from build123d import *

# Parameters (mm, degrees)
SKETCH1_R               = 6.5
SKETCH1_R_2             = 6
SKETCH1_R_3             = 5.3
BOSS_EXTRUDE1_DEPTH     = 2.5
CUT_EXTRUDE1_DEPTH      = 10.526279442
CIRPATTERN1_COUNT       = 24
CUT_EXTRUDE2_DEPTH      = 10.48407185
CUT_EXTRUDE2_DEPTH_BACK = 10.48407185
SKETCH4_R               = 1.05


with BuildPart() as part:
    # Sketch1 → Boss-Extrude1 (new, symmetric)
    # profile 1 of 3: a face of its own
    with BuildSketch(Plane(origin=(0, 0, 0), x_dir=(1, 0, 0), z_dir=(0, 1, 0))):
        with Locations(Location((0, 0, 0), (0, 0, 270))):
            Circle(SKETCH1_R)
        Circle(SKETCH1_R_2, mode=Mode.SUBTRACT)
    # profile 2 of 3: a face of its own
    with BuildSketch(Plane(origin=(0, 0, 0), x_dir=(1, 0, 0), z_dir=(0, 1, 0))):
        Circle(SKETCH1_R_2)
        Circle(SKETCH1_R_3, mode=Mode.SUBTRACT)
    # profile 3 of 3: a face of its own
    with BuildSketch(Plane(origin=(0, 0, 0), x_dir=(1, 0, 0), z_dir=(0, 1, 0))):
        Circle(SKETCH1_R_3)
    extrude(amount=BOSS_EXTRUDE1_DEPTH, both=True)

    # Sketch3 → Cut-Extrude1 (cut, symmetric)
    with BuildSketch(Plane(origin=(0, 0, 0), x_dir=(1, 0, 0), z_dir=(0, 1, 0))):
        with BuildLine():
            ThreePointArc((-2.097447593, 7.48155155), (-0.805034356, 6.699886195), (-0.253044756, 5.293955832))
            ThreePointArc((-0.253044756, 5.293955832), (0, 5.3), (0.253044756, 5.293955832))
            ThreePointArc((0.253044756, 5.293955832), (0.805034356, 6.699886195), (2.097447593, 7.48155155))
            ThreePointArc((2.097447593, 7.48155155), (0, 7.77), (-2.097447593, 7.48155155))
        make_face()
    cut_extrude1 = extrude(amount=CUT_EXTRUDE1_DEPTH, both=True, mode=Mode.SUBTRACT)

    # CirPattern1: Cut-Extrude1 ×24 about axis
    cirpattern1_axis = Axis((0, 0, 0), (0, 1, 0))
    for i in range(1, CIRPATTERN1_COUNT):
        add(cut_extrude1.rotate(cirpattern1_axis, i * 360 / CIRPATTERN1_COUNT), mode=Mode.SUBTRACT)

    # Sketch4 → Cut-Extrude2 (cut, two sides: drawn at the far end of the back side and taken through both)
    with BuildSketch(Plane(origin=(0, 0, 0), x_dir=(1, 0, 0), z_dir=(0, 1, 0)).offset(-CUT_EXTRUDE2_DEPTH_BACK)):
        with Locations(Location((0, 0, 0), (0, 0, 270))):
            Circle(SKETCH4_R)
    extrude(amount=CUT_EXTRUDE2_DEPTH + CUT_EXTRUDE2_DEPTH_BACK, mode=Mode.SUBTRACT)


solid = part.part
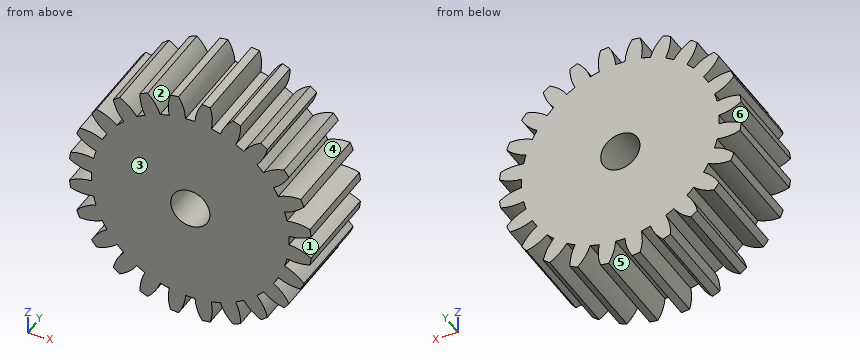
Read the model definition and answer for the solid it produces. Units are mm, in the model's axes. Face numbers are marked on the shaded views. A direction names the side the tool comes from. Round coordinates to 2 decimals unless told otherwise and drop trailing zeros. Order: outer loops, then holes, each group sorted by start corner. A loop starts at its lowest first (then second) coordinate and runs counter-clockwise, first axis right, second up.
1) The part is cut by section C-C on z = 5.5. Write down the section's boundary in (x, y), plus the area to 3 significant figures.
2) The part is cut by section A-A on z = 0. Write down the section's boundary in (x, y), plus the area to 3 significant figures.
3) The part is cut by section B-B on x = 0. Write down the section's boundary in (y, z).
4) Flat-ended cylindrical pins translate along their axes: pin 1 (1 mm diameter, centred on x = -4, y = 0.5, fed in from +Z); pin 2 (1 mm diameter, centred on y = -1, z = -1.5, fed in from +X). Find the tip coordinate at first contact, or state that the pin passes through.
5) The part is cut by section D-D on x = 5.5. Write down the section's boundary in (y, z).
6) Straight lines are drawn through the part: L1, parallel to X at y = 1.2, z = -6; L2, parallel to X at y = -1.15, z = -5; L3, parallel to Z at x = -5.5, y = 0.8. For each, find the intervals that lie inside material, in ascending order.
7) For the marked faces 4, 5 and 6, determine the directions among +Z, -Z, +X, -X, +Y, -Y from which every point of the face is accessible in a straight line to the end or side of a thin tool.
8) The mould has two halves that part along X. Classify the marked faces 1, 2 and 3: released by +X, released by -X, zero draft, split by the parting line, or undercut.
Resolved:
1. outline: (-2.67, -2.5) - (-1.81, -2.5) - (-1.81, 2.5) - (-2.67, 2.5) - close; (-1.17, -2.5) - (-0.27, -2.5) - (-0.27, 2.5) - (-1.17, 2.5) - close; (0.27, -2.5) - (1.17, -2.5) - (1.17, 2.5) - (0.27, 2.5) - close; (1.81, -2.5) - (2.67, -2.5) - (2.67, 2.5) - (1.81, 2.5) - close
1. area: 17.6 mm2
2. outline: (-5.3, -2.5) - (-1.05, -2.5) - (-1.05, 2.5) - (-5.3, 2.5) - close; (1.05, -2.5) - (5.3, -2.5) - (5.3, 2.5) - (1.05, 2.5) - close
2. area: 42.5 mm2
3. outline: (-2.5, -5.3) - (2.5, -5.3) - (2.5, -1.05) - (-2.5, -1.05) - close; (-2.5, 1.05) - (2.5, 1.05) - (2.5, 5.3) - (-2.5, 5.3) - close
4. pin 1: stops at z = 5.29
4. pin 2: stops at x = 6.42
5. outline: (-2.5, -2.67) - (2.5, -2.67) - (2.5, -1.81) - (-2.5, -1.81) - close; (-2.5, -1.17) - (2.5, -1.17) - (2.5, -0.27) - (-2.5, -0.27) - close; (-2.5, 0.27) - (2.5, 0.27) - (2.5, 1.17) - (-2.5, 1.17) - close; (-2.5, 1.81) - (2.5, 1.81) - (2.5, 2.67) - (-2.5, 2.67) - close
6. L1: x = -2.5 to -2.2, -1.16 to -0.4, 0.4 to 1.16, 2.2 to 2.5
6. L2: x = -4.12 to -3.35, -2.55 to 2.55, 3.35 to 4.12
6. L3: z = -2.67 to -1.81, -1.17 to -0.27, 0.27 to 1.17, 1.81 to 2.67
7. face 4: +Y, -Y
7. face 5: -Z, +Y, -Y
7. face 6: -X, +Y, -Y
8. face 1: released by +X
8. face 2: undercut
8. face 3: zero draft
